from build123d import *

# Parameters (mm, degrees)
F0_W     = 406.4
F0_H     = 406.4
F1_DEPTH = 88.9
F2_R     = 50.8
F3_R     = 12.7


with BuildPart() as f1:
    # F0 (on Top) → F1 (new body)
    with BuildSketch(Plane.XY):
        Rectangle(F0_W, F0_H)
    extrude(amount=-F1_DEPTH)

    # F2
    f2_edges = [f1.edges().sort_by_distance(p)[0] for p in [
        (-203.2, -203.2, -44.45),
        (203.2, -203.2, -44.45),
        (203.2, 203.2, -44.45),
        (-203.2, 203.2, -44.45),
    ]]
    fillet(f2_edges, radius=F2_R)

    # F3
    f3_edges = [f1.edges().sort_by_distance(p)[0] for p in [
        (0, 203.2, 0),
    ]]
    fillet(f3_edges, radius=F3_R)


solid = f1.part
Design review of the part built by this model. Coordinates are the model's own, in mm. Give positions to 0.01 mm unless a question says otherwise; leave off trailing zeros. Order: outer loops, then holes, each group sorted by start corner. A loop starts at its lowest first (then second) coordinate and runs counter-clockwise, first axis right, second up. Notation, with made-up numbers: (28.25, 85) - (75.25, 85) arc R30 ccw to (75.25, 116) - close; hole circle Ø11 at (70, -25). An arc over 180 degrees is marked (long way). Write item = value, one per line. Start each with the question number.
Q1. We need section A-A on z = -6. State the section outline as (x, y) points.
Q2. To check wall thickness, follow L1, parallel to Y at x = 160, z = -24; L2, parallel to X at y = 158, z = -56; L3, parallel to Y at x = -72.5, z = -10. State the ranges of each line that lie inside material, in increasing order. Write a range as from..to.
Q3. Clearance check with a flat-ended pin moving along its axis: pin 1 Ø2 at (x, z) = (157, -45) entering from -Y. State where the tip first meets the part, or that it passes through.
Working result:
q1.outline = (-201.29, -152.4) arc R48.89 ccw to (-152.4, -201.29) - (152.4, -201.29) arc R48.89 ccw to (201.29, -152.4) - (201.29, 152.4) arc R48.89 ccw to (152.4, 201.29) - (-152.4, 201.29) arc R48.89 ccw to (-201.29, 152.4) - close
q2.L1 = -202.63..202.63
q2.L2 = -202.89..202.89
q2.L3 = -202.91..202.91
q3.pin_1 = -203.07
